Read the model definition and answer for the solid it produces. Units are mm, in the model's axes. A direction names the side the tool comes from. Coordinates: 2 decimals unless noted, no trailing zeros. Order: outer loops, then holes, each group sorted by start corner. A loop starts at its lowest first (then second) coordinate and runs counter-clockwise, first axis right, second up.
from build123d import *

# Parameters (mm, degrees)
SKETCH_1_W          = 42
SKETCH_1_H          = 42
EXTRUDE_1_DEPTH     = 40
SKETCH_2_R          = 11
EXTRUDE_2_DEPTH     = 2
SKETCH_3_R          = 2.5
EXTRUDE_3_DEPTH     = 22
SKETCH_4_R          = 1.5
CUT_EXTRUDE_1_DEPTH = 4.5
CHAMFER_1_SIZE      = 5
SKETCH_5_W          = 16.42199876
SKETCH_5_H          = 2.116075979
EXTRUDE_4_DEPTH     = 7


with BuildPart() as part:
    # 草图1 → 凸台-拉伸1 (new body)
    with BuildSketch(Plane(origin=(0, 0, 0), x_dir=(1, 0, 0), z_dir=(0, 1, 0))):
        Rectangle(SKETCH_1_W, SKETCH_1_H)
    extrude(amount=EXTRUDE_1_DEPTH)

    # 草图2 → 凸台-拉伸2 (add)
    with BuildSketch(Plane(origin=(0, 40, 0), x_dir=(1, 0, 0), z_dir=(0, 1, 0))):
        with Locations(Location((0, 0, 0), (0, 0, 270))):
            Circle(SKETCH_2_R)
    extrude(amount=EXTRUDE_2_DEPTH)

    # 草图3 → 凸台-拉伸3 (add)
    with BuildSketch(Plane(origin=(0, 42, 0), x_dir=(1, 0, 0), z_dir=(0, 1, 0))):
        with Locations(Location((0, 0, 0), (0, 0, 270))):
            Circle(SKETCH_3_R)
    extrude(amount=EXTRUDE_3_DEPTH)

    # 草图4 → 切除-拉伸1 (cut)
    with BuildSketch(Plane(origin=(0, 40, 0), x_dir=(1, 0, 0), z_dir=(0, 1, 0))):
        with Locations(Location((-15.5, 15.5, 0), (0, 0, 270))):
            Circle(SKETCH_4_R)
        with Locations(Location((15.5, 15.5, 0), (0, 0, 270))):
            Circle(SKETCH_4_R)
        with Locations(Location((15.5, -15.5, 0), (0, 0, 270))):
            Circle(SKETCH_4_R)
        with Locations(Location((-15.5, -15.5, 0), (0, 0, 270))):
            Circle(SKETCH_4_R)
    extrude(amount=-CUT_EXTRUDE_1_DEPTH, mode=Mode.SUBTRACT)

    # 倒角1
    chamfer_1_edges = [part.edges().sort_by_distance(p)[0] for p in [
        (21, 20, 21),
        (-21, 20, 21),
        (-21, 20, -21),
        (21, 20, -21),
    ]]
    chamfer(chamfer_1_edges, length=CHAMFER_1_SIZE)

    # 草图5 → 凸台-拉伸4 (add)
    with BuildSketch(Plane.ZY.offset(21)):
        with Locations((0, 1.05803799)):
            Rectangle(SKETCH_5_W, SKETCH_5_H)
    extrude(amount=EXTRUDE_4_DEPTH)


solid = part.part
Q1. Straight lines are drawn through the part: L1, parallel to X at y = 37, z = 15.5; L2, parallel to Z at x = -15, y = 38. For each, find the intervals that lie inside material, in ascending order.
Q2. The part is cut by section B-B, the plane x = 0. Determine the outline of the cut face in (y, z).
Q3. Each of these flat-tipped pins is pushed along its axis until it touches: P1, Ø12, axis at x = -19.5, z = -14, coming from the +Y side; P2, Ø1.7, axis at x = -25, y = 1, coming from the +Z side; P3, Ø2, axis at x = -23, z = 1, coming from the +Y side. Where does it stop, or does it pass through?
Q4. The part is cut by section A-A, the plane y = 34.5. Determine the outline of the cut face in (x, z), then the cut area to 3 significant figures.
Q5. Which of the six approach directions +Z, -Z, +X, -X, +Y, -Y give full straight-line access (tool end or side, diameter ignored) to faces 1 (the cylindrical face through (-15.43, 37.78, 14)), 2 (the flat face through (-24, 2.116, 0)), 3 (the flat face through (-24, 1, -8.211)), 4 (the flat face through (19, 20, 18)), 5 (the flat face through (-24, 1, 8.211))?
Q6. The part is cut by section C-C, the plane z = 0. Determine the outline of the cut face in (x, y), then the cut area to 3 significant figures.
Q7. The part is cut by section D-D, the plane x = -6.5. Determine the outline of the cut face in (y, z), then the cut area to 3 significant figures.
Q8. Determine the mould class of faces 6 (the flat face through (0, 20, 21)), 7 (the flat face through (-15, 35.5, -16)), 8 (the flat face through (-18, 20, 19)), 9 (the flat face through (16, 35.5, 15)) for opening direction X: +X half, -X half, draft (parallel to the pull), parting line (faces both ways), or undercut.
Computed values:
1. L1: x = -21 to -17, -14 to 14, 17 to 21
1. L2: z = -21 to -16.91, -14.09 to 14.09, 16.91 to 21
2. outline: (0, -21) - (40, -21) - (40, -11) - (42, -11) - (42, -2.5) - (64, -2.5) - (64, 2.5) - (42, 2.5) - (42, 11) - (40, 11) - (40, 21) - (0, 21) - close
3. P1: stops at y = 40
3. P2: stops at z = 8.21
3. P3: stops at y = 2.12
4. outline: (-21, -16) - (-16, -21) - (16, -21) - (21, -16) - (21, 16) - (16, 21) - (-16, 21) - (-21, 16) - close
4. area: 1,710 mm2
5. face 1: +Y
5. face 2: +Z, -Z, -X, +Y
5. face 3: -Z, -X, +Y, -Y
5. face 4: +Z, +X, +Y, -Y
5. face 5: +Z, -X, +Y, -Y
6. outline: (-28, 0) - (21, 0) - (21, 40) - (11, 40) - (11, 42) - (2.5, 42) - (2.5, 64) - (-2.5, 64) - (-2.5, 42) - (-11, 42) - (-11, 40) - (-21, 40) - (-21, 2.12) - (-28, 2.12) - close
6. area: 1,850 mm2
7. outline: (0, -21) - (40, -21) - (40, -8.87) - (42, -8.87) - (42, 8.87) - (40, 8.87) - (40, 21) - (0, 21) - close
7. area: 1,720 mm2
8. face 6: draft
8. face 7: undercut
8. face 8: -X half
8. face 9: undercut
